For this review, use the dimensioned drawing (mm, ordinates from the lowest corner) and the shaded views. Give positions to 0.01 mm unless a question says otherwise; leave off trailing zeros. Loops run counter-clockwise (first coordinate to the right, second up) from the corner with the lowest first, then second, coordinate; pieces in that order, holes last. Notation, with made-up numbers: (87, 10) -> (111, 10) arc R34 ccw to (111, 49) -> close; hole circle Ø10 at (-14, 58). An arc over 180 degrees is marked (long way). Use a Markdown table: item, result. Add a question column.
1. Add section C-C (x = 8.75). State the section outline as (y, z) points, and give its area (3 significant figures).
2. For pin 1 Ø3 at (y, z) = (5, 5) entering from -X (3 decimals); pin 2 Ø1.5 at (x, y) = (5, 5) entering from -Z; pin 3 Ø1 at (x, y) = (4, 5) entering from -Z (3 decimals), all flat-tipped, find the tip position at first contact; note any pin that passes through.
3. Add section A-A (x = 5). State the section outline as (y, z) points (3 decimals).
4. To check wall thickness, follow line 1 (Y direction, x = 5, z = 2.2); line 2 (X direction, y = 1, z = 5.75). State the ranges of each line that lie inside material, in increasing order.
5. Draft analysis for pull direction Z (two halves, no side actions). For the marked faces 1, 2 and 3, state which applies: pulls with the +Z half, pulls with the -Z half, needs draft (parallel to the pull), parting line crosses it, or undercut.
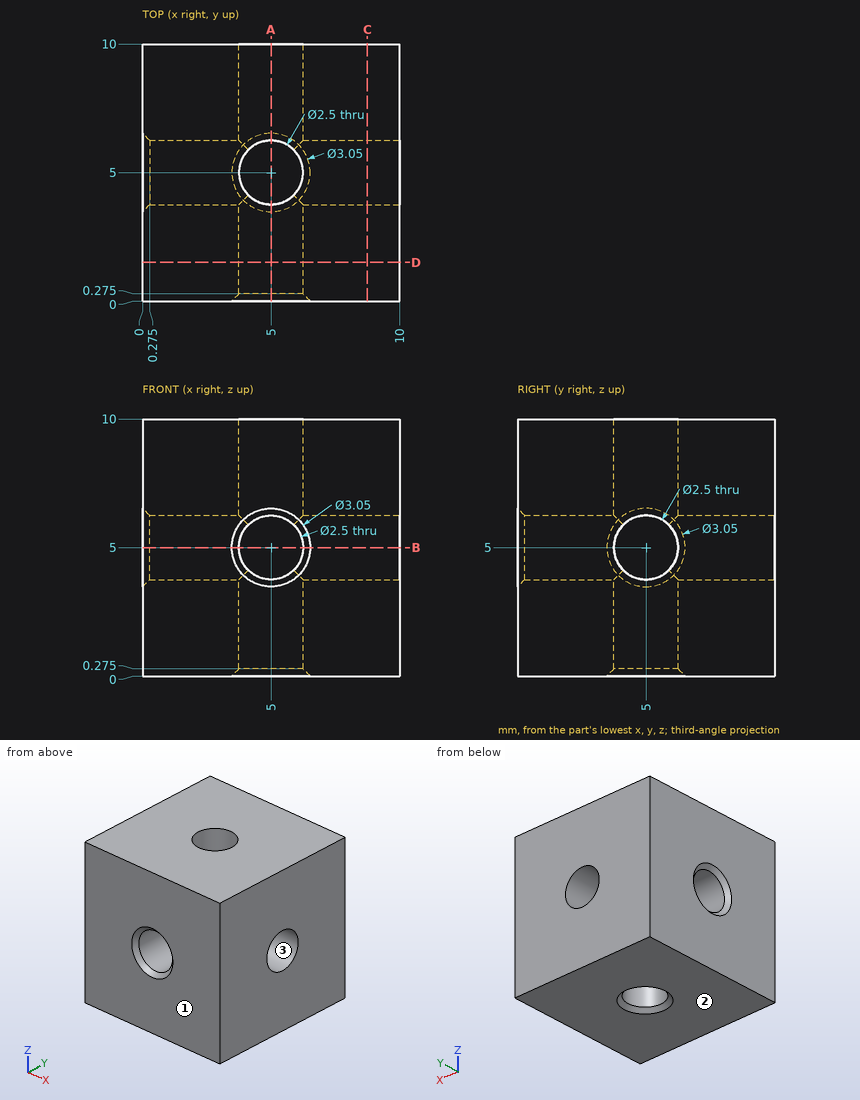
Taken from the geometry:
| question | item | result |
|---|---|---|
| 1 | outline | (0, 0) -> (10, 0) -> (10, 10) -> (0, 10) -> close; hole circle Ø2.5 at (5, 5) |
| 1 | area | 95.1 mm^2 |
| 2 | pin 1 | stops at x = 0.025 |
| 2 | pin 2 | passes through |
| 2 | pin 3 | stops at z = 0.025 |
| 3 | outline | (0, 0) -> (3.475, 0) -> (3.75, 0.275) -> (3.75, 3.75) -> (0.275, 3.75) -> (0, 3.475) -> close; (0, 6.525) -> (0.275, 6.25) -> (3.75, 6.25) -> (3.75, 10) -> (0, 10) -> close; (6.25, 0.275) -> (6.525, 0) -> (10, 0) -> (10, 3.75) -> (6.25, 3.75) -> close; (6.25, 6.25) -> (10, 6.25) -> (10, 10) -> (6.25, 10) -> close |
| 4 | line 1 | y = 0 to 3.75, 6.25 to 10 |
| 4 | line 2 | x = 0 to 4, 6 to 10 |
| 5 | face 1 | needs draft |
| 5 | face 2 | pulls with the -Z half |
| 5 | face 3 | undercut |
